from build123d import *

# Parameters (mm, degrees)
SKETCH1_W           = 66.16
SKETCH1_H           = 6
BOSS_EXTRUDE1_DEPTH = 3.175
SKETCH3_W           = 4.8
SKETCH3_H           = 0.9
CUT_EXTRUDE1_DEPTH  = 34.367154883
FILLET1_R           = 0.8
FILLET2_R           = 0.1


with BuildPart() as part:
    # Sketch1 → Boss-Extrude1 (new body)
    with BuildSketch(Plane.XY):
        Rectangle(SKETCH1_W, SKETCH1_H)
    extrude(amount=BOSS_EXTRUDE1_DEPTH)

    # Sketch3 → Cut-Extrude1 (cut, through all)
    with BuildSketch(Plane.XY.offset(3.175)):
        with Locations((-30.68, 2.55)):
            Rectangle(SKETCH3_W, SKETCH3_H)
        with Locations((-30.68, -2.55)):
            Rectangle(SKETCH3_W, SKETCH3_H)
    cut_extrude1 = extrude(amount=-CUT_EXTRUDE1_DEPTH, mode=Mode.SUBTRACT)

    # Mirror1: Cut-Extrude1 across plane
    add(cut_extrude1.mirror(Plane(origin=(0, 0, 0), x_dir=(0, 0, 1), z_dir=(1, 0, 0))), mode=Mode.SUBTRACT)

    # Fillet1
    fillet1_edges = [part.edges().sort_by_distance(p)[0] for p in [
        (-33.08, 2.1, 1.5875),
        (-33.08, -2.1, 1.5875),
        (33.08, 2.1, 1.5875),
        (33.08, -2.1, 1.5875),
    ]]
    fillet(fillet1_edges, radius=FILLET1_R)

    # Fillet2
    fillet2_edges = [part.edges().sort_by_distance(p)[0] for p in [
        (-28.28, 3, 1.5875),
        (-28.28, 2.1, 1.5875),
        (-28.28, -2.1, 1.5875),
        (-28.28, -3, 1.5875),
        (28.28, 2.1, 1.5875),
        (28.28, 3, 1.5875),
        (28.28, -3, 1.5875),
        (28.28, -2.1, 1.5875),
    ]]
    fillet(fillet2_edges, radius=FILLET2_R)


solid = part.part
Model file for the job. Use its own axes, mm. A direction names the side the tool comes from. Give positions to 0.01 mm unless a question says otherwise; leave off trailing zeros. Order: outer loops, then holes, each group sorted by start corner. A loop starts at its lowest first (then second) coordinate and runs counter-clockwise, first axis right, second up. Notation, with made-up numbers: M 88.5,89 L 146.5,89 A23 ccw 146.5,119 Z; hole C -0.5,0 d5. An arc over 180 degrees is marked long. Write item = value, one per line.
Q1. Tool access for faces 1 (the flat face through (30, -2.1, 2)), 2 (the flat face through (-30, 2.1, 2)), 3 (the flat face through (30, 2.1, 2)): list every direction of +Z, -Z, +X, -X, +Y, -Y with a clear straight run to the whole face (end or side of a thin tool).
Derived:
face_1 = +Z, -Z, +X, -Y
face_2 = +Z, -Z, -X, +Y
face_3 = +Z, -Z, +X, +Y
Q2. Drill centre lines: line 1 (X direction, y = -2.3, z = 0.35); line 2 (X direction, y = 1.7, z = 0.65). Where is each one in solid material? Low to high. Write a range as [from, to].
Derived:
line_1 = [-28.28, 28.28]
line_2 = [-32.97, 32.97]
Q3. Flat gauge pins, fed straight in: pin 1 (1 mm diameter, centred on x = -31, z = 1.5, fed in from +Y); pin 2 (1.6 mm diameter, centred on x = -31, z = 2.5, fed in from -Y). Where does each tip first touch, or does it go through?
Derived:
pin_1 = 2.1
pin_2 = -2.1
Q4. Cut at A-A, the plane z = 1.5. List the corners of the cut face in (x, y), then the cut area to 3 significant figures.
Derived:
outline = M -33.08,-1.3 A0.8 ccw -32.28,-2.1 L -28.38,-2.1 A0.1 cw -28.28,-2.2 L -28.28,-2.9 A0.1 ccw -28.18,-3 L 28.18,-3 A0.1 ccw 28.28,-2.9 L 28.28,-2.2 A0.1 cw 28.38,-2.1 L 32.28,-2.1 A0.8 ccw 33.08,-1.3 L 33.08,1.3 A0.8 ccw 32.28,2.1 L 28.38,2.1 A0.1 cw 28.28,2.2 L 28.28,2.9 A0.1 ccw 28.18,3 L -28.18,3 A0.1 ccw -28.28,2.9 L -28.28,2.2 A0.1 cw -28.38,2.1 L -32.28,2.1 A0.8 ccw -33.08,1.3 Z
area = 379 mm2
